Check sheet for the modelled part. Datum: model origin and axes. Units: mm. Round coordinates to 2 decimals unless told otherwise and drop trailing zeros. Order: outer loops, then holes, each group sorted by start corner. A loop starts at its lowest first (then second) coordinate and runs counter-clockwise, first axis right, second up.
Q1. Cross-section at A-A on y = 24.5. Record the cut outline in (x, z), then the cut area to 3 significant figures.
Q2. Scan lines: probe 1 along Y at (x, z) = (9, 18.75); probe 2 along Y at (x, z) = (-1, 8); probe 3 along X at (y, z) = (26.5, 18.75). Record each from-to range of solid material in increasing order.
Q3. Depth check by flat-ended pin: P1, Ø4, axis at y = -30, z = 18.5, coming from the -X side; P2, Ø6, axis at x = 25, z = 3, coming from the -Y side. Enter the tip coordinate at first touch or a pass-through.
Q4. Cross-section at C-C on z = 13. Give the number of separate pieces and of enclosed holes in the cut face, then the cut area to 3 significant figures.
Q5. Mould release check, pull along X, two halves, no side actions. Record for faces 1 (the cylindrical face through (0.97, 41.48, 12.88)), 2 (the cylindrical face through (29.06, 47.2, 12.88)), 3 (the flat face through (5, -1, 25.4)), 4 (the cylindrical face through (-18.76, 47.12, 12.88)): +X half, -X half, draft (parallel to the pull), parting line (faces both ways), or undercut.
Q6. Cross-section at B-B on x = 2.5. Record the cut outline in (y, z), then the cut area to 3 significant figures.
Q7. Cross-section at D-D on x = -4.5. Record the cut outline in (y, z).
from build123d import *

# Parameters (mm, degrees)
F0_W     = 50.8
F0_H     = 101.6
F1_DEPTH = 25.4
F2_R     = 12.7
F3_DEPTH = 131
F4_D     = 25.4
F6_D     = 25.4
F7_R     = 25.39999
F8_R     = 5.08


# Not quite as in the source:
# - a fillet or chamfer is up to 0.001 mm smaller than in the source, because OpenCascade refuses the exact size
# - an extrude ends at something that could not be found from the text; its depth is read off the source's solid


with BuildPart() as f1:
    # F0 (on Top) → F1 (new body)
    with BuildSketch(Plane.XY):
        with Locations((5.1918309937, -2.1536122621)):
            Rectangle(F0_W, F0_H)
    extrude(amount=F1_DEPTH)

    # F2 (on Top) → F3 (cut, through all)
    with BuildSketch(Plane.XY):
        with Locations((4.7334181145, -35.6077803201)):
            Circle(F2_R)
    extrude(amount=-F3_DEPTH, mode=Mode.SUBTRACT)

    # F4 (through all)
    with Locations(Plane(origin=(0, 0, 0), x_dir=(1, 0, 0), z_dir=(0, 0, -1))):
        with Locations((4.7334181145, 35.6077803201)):
            Hole(F4_D / 2)

    # F6 (through all)
    with Locations(Plane(origin=(0, 0, 0), x_dir=(1, 0, 0), z_dir=(0, 0, -1))):
        with Locations((6.8339584395, -30.2138105035)):
            Hole(F6_D / 2)

    # F7 (radius 25.4 in the source; OpenCascade refuses exactly that, so slightly less here)
    f7_edges = [f1.edges().sort_by_distance(p)[0] for p in [
        (-20.208169, -52.953612, 12.7),
        (30.591831, -52.953612, 12.7),
    ]]
    fillet(f7_edges, radius=F7_R)

    # F8
    f8_edges = [f1.edges().sort_by_distance(p)[0] for p in [
        (-20.208169, 48.646388, 12.7),
        (30.591831, 48.646388, 12.7),
    ]]
    fillet(f8_edges, radius=F8_R)


solid = f1.part
Results found:
1. outline: (-20.21, 0) - (-4.51, 0) - (-4.51, 25.4) - (-20.21, 25.4) - close; (18.18, 0) - (30.59, 0) - (30.59, 25.4) - (18.18, 25.4) - close
1. area: 714 mm2
2. probe 1: y = -52.67 to -47.57, -23.65 to 17.7, 42.73 to 48.65
2. probe 2: y = -52.19 to -46.94, -24.28 to 20.22, 40.21 to 48.65
2. probe 3: x = -20.21 to -5.31, 18.98 to 30.59
3. P1: stops at x = -20.2
3. P2: stops at y = -46.6
4. separate pieces: 1
4. enclosed holes: 2
4. area: 3,860 mm2
5. face 1: undercut
5. face 2: +X half
5. face 3: draft
5. face 4: -X half
6. outline: (-52.81, 0) - (-48.11, 0) - (-48.11, 25.4) - (-52.81, 25.4) - close; (-23.11, 0) - (18.28, 0) - (18.28, 25.4) - (-23.11, 25.4) - close; (42.15, 0) - (48.65, 0) - (48.65, 25.4) - (42.15, 25.4) - close
6. area: 1,340 mm2
7. outline: (-51.03, 0) - (-44.33, 0) - (-44.33, 25.4) - (-51.03, 25.4) - close; (-26.89, 0) - (24.48, 0) - (24.48, 25.4) - (-26.89, 25.4) - close; (35.94, 0) - (48.65, 0) - (48.65, 25.4) - (35.94, 25.4) - close
